from build123d import *

# Parameters (mm, degrees)
F0_R     = 4.7625
F1_DEPTH = 12.7
F2_R     = 46.355
F2_R_2   = 33.655
F3_DEPTH = 88.9
F4_R     = 2.54


with BuildPart() as f1:
    # F0 (on Top) → F1 (new body)
    with BuildSketch(Plane.XY):
        with BuildLine():
            ThreePointArc((53.975, 41.275), (50.255256, 50.255256), (41.275, 53.975))
            Line((41.275, 53.975), (-41.275, 53.975))
            ThreePointArc((-41.275, 53.975), (-50.255256, 50.255256), (-53.975, 41.275))
            Line((-53.975, 41.275), (-53.975, -41.275))
            ThreePointArc((-53.975, -41.275), (-50.255256, -50.255256), (-41.275, -53.975))
            Line((-41.275, -53.975), (41.275, -53.975))
            ThreePointArc((41.275, -53.975), (50.255256, -50.255256), (53.975, -41.275))
            Line((53.975, -41.275), (53.975, 41.275))
        make_face()
        with Locations((-41.275, -41.275)):
            Circle(F0_R, mode=Mode.SUBTRACT)
        with Locations((41.275, -41.275)):
            Circle(F0_R, mode=Mode.SUBTRACT)
        with Locations((-41.275, 41.275)):
            Circle(F0_R, mode=Mode.SUBTRACT)
        with Locations((41.275, 41.275)):
            Circle(F0_R, mode=Mode.SUBTRACT)
    extrude(amount=F1_DEPTH)

    # F2 (on face) → F3 (join)
    with BuildSketch(Plane.XY.offset(12.7)):
        Circle(F2_R)
        Circle(F2_R_2, mode=Mode.SUBTRACT)
    extrude(amount=F3_DEPTH)

    # F4
    f4_edges = [f1.edges().sort_by_distance(p)[0] for p in [
        (-46.355, 0, 12.7),
        (0, -53.975, 12.7),
        (-46.355, 0, 101.6),
    ]]
    fillet(f4_edges, radius=F4_R)


solid = f1.part
The listing builds one solid part. Answer for the finished solid, in the listing's coordinates (mm). A direction names the side the tool comes from. Coordinates: 2 decimals unless noted, no trailing zeros. Order: outer loops, then holes, each group sorted by start corner. A loop starts at its lowest first (then second) coordinate and runs counter-clockwise, first axis right, second up. Notation, with made-up numbers: (34, -17) -> (61, -17) arc R8 ccw to (61, -2) -> close; hole circle Ø1 at (2, 18.25). An arc over 180 degrees is marked (long way). Answer in a Markdown table with one row per item. Add a question column.
Item 1: Find the intervals of material crossed by L1, parallel to Y at x = 0, z = 38 (3 decimals); L2, parallel to Z at x = 4, y = 15; L3, parallel to Y at x = 23.5, z = 44, in increasing order. Write a range as from..to.
Item 2: Find section C-C (z = 85.5). Write down the section's boundary in (x, y) (3 decimals), then the cut area to 3 significant figures.
Item 3: Each of these flat-tipped pins is pushed along its axis until it touches: P1, Ø4, axis at x = 38.5, z = 88.5, coming from the -Y side; P2, Ø5, axis at x = -27.5, z = 32.5, coming from the +Y side; P3, Ø4, axis at x = 13.5, z = 46, coming from the +Y side. Where does it stop, or does it pass through?
Item 4: Which of the six approach directions +Z, -Z, +X, -X, +Y, -Y give full straight-line access (tool end or side, diameter ignored) to faces 1 (the face through (-39.08, 37.05, 6.26)), 2 (the face through (-7.296, -32.855, 56.528))?
Item 5: Find section A-A (y = 0). Write down the section's boundary in (x, z) (3 decimals), then the cut area to 3 significant figures.
Result set:
| question | item | result |
|---|---|---|
| 1 | L1 | y = -46.355..-33.655, 33.655..46.355 |
| 1 | L2 | z = 0..12.7 |
| 1 | L3 | y = -39.96..-24.09, 24.09..39.96 |
| 2 | outline | circle Ø92.71 at (0, 0); hole circle Ø67.31 at (0, 0) |
| 2 | area | 3,190 mm² |
| 3 | P1 | stops at y = -28.58 |
| 3 | P2 | stops at y = 39.04 |
| 3 | P3 | stops at y = 44.91 |
| 4 | face 1 | +Z, -Z |
| 4 | face 2 | +Z |
| 5 | outline | (-53.975, 0) -> (53.975, 0) -> (53.975, 10.16) arc R2.54 ccw to (51.435, 12.7) -> (48.895, 12.7) arc R2.54 cw to (46.355, 15.24) -> (46.355, 99.06) arc R2.54 ccw to (43.815, 101.6) -> (33.655, 101.6) -> (33.655, 12.7) -> (-33.655, 12.7) -> (-33.655, 101.6) -> (-43.815, 101.6) arc R2.54 ccw to (-46.355, 99.06) -> (-46.355, 15.24) arc R2.54 cw to (-48.895, 12.7) -> (-51.435, 12.7) arc R2.54 ccw to (-53.975, 10.16) -> close |
| 5 | area | 3,630 mm² |
